Source: CAD feature listing. Evaluate the final solid. Frame: model axes, mm. Face numbers are marked on the shaded views. A direction names the side the tool comes from. Round coordinates to 2 decimals unless told otherwise and drop trailing zeros. Loops run counter-clockwise (first coordinate to the right, second up) from the corner with the lowest first, then second, coordinate; pieces in that order, holes last. Notation, with made-up numbers: (88, 13) -> (109, 13) arc R23 cw to (109, 23) -> close; hole circle Ø2 at (71, 28.5). An arc over 180 degrees is marked (long way). Put each result on its own line as item: value. Start each with the question number.
1. Cut plane B-B (y = 247.5). Return the cut outline in (x, z), then the cut area to 3 significant figures.
2. Material intervals for L1, parallel to X at y = 329, z = -82; L2, parallel to X at y = 24, z = -60; L3, parallel to Z at x = 65, y = 319.5, sorted ascending.
3. Cut plane A-A (y = 195). Return the cut outline in (x, z), then the cut area to 3 significant figures.
4. Set-up query: the marked faces 1, 2 and 3. Return all of +Z, -Z, +X, -X, +Y, -Y with unobstructed straight access to the full face (end or side cutting, diameter ignored); none if empty.
5. Draft query along Y for the marked faces 4, 5, 6 and 7. Return one class per face: pulls with the +Y half, pulls with the -Y half, needs draft (parallel to the pull), parting line crosses it, or undercut.
6. Contact query for flat-ended pins moving along their axis: pin 1 (2 mm diameter, centred on y = 299, z = -65.5, fed in from +X); pin 2 (15 mm diameter, centred on x = 51.5, y = 27, fed in from +Z); pin 3 (6 mm diameter, centred on y = 83.5, z = -105, fed in from +X). Output: stop coordinate, or through.
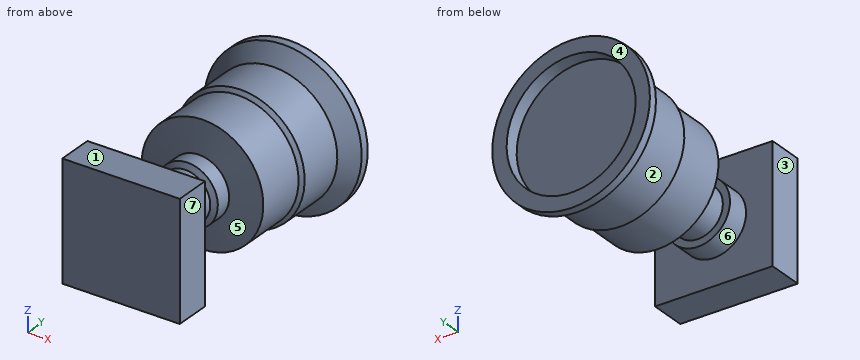
```python
from build123d import *

# Parameters (mm, degrees)
SKETCH1_W           = 164
SKETCH1_H           = 164
BOSS_EXTRUDE1_DEPTH = 50
SKETCH2_R           = 45
BOSS_EXTRUDE2_DEPTH = 32
SKETCH3_R           = 35
BOSS_EXTRUDE3_DEPTH = 45
SKETCH4_R           = 42.5
BOSS_EXTRUDE4_DEPTH = 25
SKETCH5_R           = 85
BOSS_EXTRUDE5_DEPTH = 80
SKETCH6_R           = 90
BOSS_EXTRUDE6_DEPTH = 70
SKETCH7_R           = 110
BOSS_EXTRUDE7_DEPTH = 32
CHAMFER1_SIZE       = 20
CHAMFER2_SIZE       = 5
CHAMFER3_SIZE       = 10
CHAMFER3_SIZE_2     = 56.712818196
CHAMFER4_SIZE       = 5
CHAMFER4_SIZE_2     = 8.660254038
CUT_EXTRUDE1_START  = -20
SKETCH8_R           = 90
CUT_EXTRUDE1_DEPTH  = 20


# Some blends are built 0.0001 mm under size
with BuildPart() as part:
    # Sketch1 → Boss-Extrude1 (new body)
    with BuildSketch(Plane(origin=(0, 0, 0), x_dir=(1, 0, 0), z_dir=(0, 1, 0))):
        with Locations((82, 82)):
            Rectangle(SKETCH1_W, SKETCH1_H)
    extrude(amount=BOSS_EXTRUDE1_DEPTH)

    # Sketch2 → Boss-Extrude2 (add)
    with BuildSketch(Plane(origin=(0, 50, 0), x_dir=(1, 0, 0), z_dir=(0, 1, 0))):
        with Locations(Location((82, 82, 0), (0, 0, 270))):
            Circle(SKETCH2_R)
    extrude(amount=BOSS_EXTRUDE2_DEPTH)

    # Sketch3 → Boss-Extrude3 (add)
    with BuildSketch(Plane(origin=(0, 82, 0), x_dir=(1, 0, 0), z_dir=(0, 1, 0))):
        with Locations(Location((82, 82, 0), (0, 0, 90))):
            Circle(SKETCH3_R)
    extrude(amount=BOSS_EXTRUDE3_DEPTH)

    # Sketch4 → Boss-Extrude4 (add)
    with BuildSketch(Plane(origin=(0, 127, 0), x_dir=(1, 0, 0), z_dir=(0, 1, 0))):
        with Locations(Location((82, 82, 0), (0, 0, 270))):
            Circle(SKETCH4_R)
    extrude(amount=BOSS_EXTRUDE4_DEPTH)

    # Sketch5 → Boss-Extrude5 (add)
    with BuildSketch(Plane(origin=(0, 152, 0), x_dir=(1, 0, 0), z_dir=(0, 1, 0))):
        with Locations(Location((82, 82, 0), (0, 0, 270))):
            Circle(SKETCH5_R)
    extrude(amount=BOSS_EXTRUDE5_DEPTH)

    # Sketch6 → Boss-Extrude6 (add)
    with BuildSketch(Plane(origin=(0, 232, 0), x_dir=(1, 0, 0), z_dir=(0, 1, 0))):
        with Locations(Location((82, 82, 0), (0, 0, 270))):
            Circle(SKETCH6_R)
    extrude(amount=BOSS_EXTRUDE6_DEPTH)

    # Sketch7 → Boss-Extrude7 (add)
    with BuildSketch(Plane(origin=(0, 302, 0), x_dir=(1, 0, 0), z_dir=(0, 1, 0))):
        with Locations(Location((82, 82, 0), (0, 0, 270))):
            Circle(SKETCH7_R)
    extrude(amount=BOSS_EXTRUDE7_DEPTH)

    # Chamfer1
    chamfer1_edges = [part.edges().sort_by_distance(p)[0] for p in [
        (82, 302, -192),
    ]]
    chamfer(chamfer1_edges, length=CHAMFER1_SIZE - 0.0001)  # a hair under: the kernel refuses the full size

    # Chamfer2
    chamfer2_edges = [part.edges().sort_by_distance(p)[0] for p in [
        (82, 232, -172),
    ]]
    chamfer(chamfer2_edges, length=CHAMFER2_SIZE - 0.0001)  # a hair under: the kernel refuses the full size

    # Chamfer3
    # the kernel refuses this chamfer: 56.712818196, 10 mm, written as the material it takes off along each edge
    with BuildSketch(Plane(origin=(82, 152, -82), x_dir=(0, 0, 1), z_dir=(-1, 0, 0))) as chamfer3_piece_1_section:
        Polygon((85, CHAMFER3_SIZE), (85 - CHAMFER3_SIZE_2, 0), (85, 0), align=None)
    chamfer3_piece_1 = revolve(axis=Axis((82, 152, -82), (0, 1, 0)), mode=Mode.PRIVATE)
    chamfer3_piece_1 = chamfer3_piece_1 - Plane(origin=(82, 157.937254532, -82), x_dir=(0, 0, 1), z_dir=(0, -1, 0)) * Cylinder(42.5, 340, mode=Mode.PRIVATE)
    add(chamfer3_piece_1, mode=Mode.SUBTRACT)

    # Chamfer4
    # the kernel refuses this chamfer: 8.660254038, 5 mm, written as the material it takes off along each edge
    with BuildSketch(Plane(origin=(82, 127, -82), x_dir=(0, 0, 1), z_dir=(-1, 0, 0))) as chamfer4_piece_1_section:
        Polygon((42.5, CHAMFER4_SIZE), (42.5 - CHAMFER4_SIZE_2, 0), (42.5, 0), align=None)
    chamfer4_piece_1 = revolve(axis=Axis((82, 127, -82), (0, 1, 0)), mode=Mode.PRIVATE)
    chamfer4_piece_1 = chamfer4_piece_1 - Plane(origin=(82, 129.764704239, -82), x_dir=(0, 0, -1), z_dir=(0, -1, 0)) * Cylinder(35, 170, mode=Mode.PRIVATE)
    add(chamfer4_piece_1, mode=Mode.SUBTRACT)

    # Sketch8 → Cut-Extrude1 (cut)
    with BuildSketch(Plane(origin=(0, 334, 0), x_dir=(1, 0, 0), z_dir=(0, 1, 0)).offset(CUT_EXTRUDE1_START)):
        with Locations(Location((82, 82, 0), (0, 0, 270))):
            Circle(SKETCH8_R)
    extrude(amount=CUT_EXTRUDE1_DEPTH, mode=Mode.SUBTRACT)


solid = part.part
```
Solution:
1. outline: circle Ø180 at (82, -82)
1. area: 25,400 mm^2
2. L1: x = -28 to -8, 172 to 192
2. L2: x = 0 to 164
2. L3: z = -188.15 to -170.38, 6.38 to 24.15
3. outline: circle Ø170 at (82, -82)
3. area: 22,700 mm^2
4. face 1: +Z, +X, -X, -Y
4. face 2: none
4. face 3: +Z, -Z, -X, -Y
5. face 4: pulls with the +Y half
5. face 5: undercut
5. face 6: undercut
5. face 7: needs draft
6. pin 1: stops at x = 170.66
6. pin 2: stops at z = 0
6. pin 3: stops at x = 122.11
